Autodesk Inventor part; units mm, degrees
ref_plane "YZ Plane" through (0, 0, 0) normal (1, 0, 0) x (0, 1, 0)
ref_plane "XZ Plane" through (0, 0, 0) normal (0, 1, 0) x (-1, 0, 0)
ref_plane "XY Plane" through (0, 0, 0) normal (0, 0, 1) x (1, 0, 0)
sketch "Sketch1" plane through (0, 0, 0) normal (0, 1, 0) x (-1, 0, 0)
  line L0 (0, 0) -> (0, 28)
  line L1 (0, 28) -> (0, 23)
  circle A0 centre (5, 23) radius 1.5
  circle A1 centre (68, 23) radius 1.5
  line L2 (0, 28) -> (71.7701, 28)
  line L3 (71.7701, 28) -> (71.7701, 0)
  line L4 (71.7701, 0) -> (0, 0)
  line L5 (0, 0) -> (0, -28)
  line L6 (0, -28) -> (0, -23)
  line L7 (0, -23) -> (5, -23)
  circle A2 centre (5, -23) radius 1.5
  circle A3 centre (68, -23) radius 1.5
  line L8 (0, -28) -> (71.7701, -28)
  line L9 (71.7701, -28) -> (71.7701, 0)
  dimension "d0" = 28
  dimension "d4" = 3
  dimension "d6" = 3
extrude "Extrusion1" add sketch "Sketch1" along normal blind 3.175
sketch "Sketch2" plane through (0, 3.175, 0) normal (0, 1, 0) x (1, 0, 0)
  line L0 (0, 28) -> (-71.7701, 28)
  line L1 (-10.8543, 28) -> (-10.8543, -28)
  line L2 (-71.7701, -28) -> (0, -28)
  line L3 (-10.8543, -28) -> (-40.8543, -28)
  line L4 (-40.8543, -28) -> (-40.8543, 28)
  line L5 (-40.8543, 28) -> (-10.8543, 28)
  line L6 (-40.8543, -28) -> (-47.2043, -28)
  line L7 (-47.2043, -28) -> (-47.2043, 28)
  line L8 (-40.8543, 28) -> (-47.2043, 28)
  point P0 (0, 0)
  dimension "d9" = 30
  dimension "d10" = 6.35
revolve "Revolution1" add sketch "Sketch2" angle 20 about axis through (-47.2043, 3.175, 28) along (0, 0, 1)
sketch "Sketch3" plane through (-47.2043, 3.175, 28) normal (-0.342, 0.9397, 0) x (0.9397, 0.342, 0)
  line L0 (0, 0) -> (0, 56)
  line L1 (0, 56) -> (6.35, 56)
  line L2 (43.2716, 56) -> (-24.1703, 56)
  line L3 (6.35, 56) -> (6.35, 0)
  line L4 (0, 0) -> (36.35, 0)
  line L5 (-23.0843, 0) -> (0, 0)
  line L6 (6.35, 0) -> (0, 0)
  line L7 (0, 0) -> (0, 56)
  point P0 (43.2716, 28)
  dimension "d12" = 6.35
extrude "Extrusion2" add sketch "Sketch3" along normal blind 44
sketch "Sketch4" plane through (0, 3.175, 0) normal (0, 1, 0) x (1, 0, 0)
  line L0 (-10.8543, 28) -> (-10.8543, -28)
  line L1 (-10.8543, 0) -> (-10.8543, -7.5)
  line L2 (-10.8543, -7.5) -> (-13.8543, -7.5)
  line L3 (-13.8543, -7.5) -> (-13.8543, 0)
  line L4 (-13.8543, 0) -> (-13.8543, 7.5)
  line L5 (-13.8543, 7.5) -> (-10.8543, 7.5)
  line L6 (-10.8543, 7.5) -> (-10.8543, 0)
  point P0 (0, 0)
  dimension "d15" = 7.5
  dimension "d16" = 3
  dimension "d17" = 7.5
extrude "Extrusion3" cut sketch "Sketch4" along normal mid plane 6.35
sketch "Sketch5" plane through (0, 3.175, 0) normal (0, 1, 0) x (1, 0, 0)
  line L0 (0, 28) -> (-10.8543, 28)
  line L1 (0, 28) -> (-53, 28)
  line L2 (0, 28) -> (-71.7701, 28)
  line L3 (-53, 0) -> (-53, 7.5)
  line L4 (-53, 7.5) -> (-56, 7.5)
  line L5 (-56, 7.5) -> (-56, 0)
  line L6 (-56, 0) -> (-56, -7.5)
  line L7 (-56, -7.5) -> (-53, -7.5)
  line L8 (-53, -7.5) -> (-53, 0)
  point P0 (0, 0)
  dimension "d20" = 53
  dimension "d21" = 7.5
  dimension "d22" = 3
  dimension "d23" = 7.5
extrude "Extrusion4" cut sketch "Sketch5" against normal blind 6.35
fillet "Fillet1" radius 3.175 8 edges at (0, 3.175, 0) (-54.7287, 23.8482, 28) (-54.7287, 23.8482, -28) (-62.2532, 44.5215, 0) (-56, 3.175, 0) (-53, 3.175, 0) (-54.5, 3.175, -7.5) (-54.5, 3.175, 7.5)
fillet "Fillet2" radius 1.524 1 edges at (-71.7701, 3.175, 0)
sketch "Sketch6" plane through (-41.2373, 5.3468, 28) normal (0.9397, 0.342, 0) x (0, 0, -1)
  line L0 (0, 44) -> (3.175, 40.825)
  line L1 (52.825, 40.825) -> (56, 44)
  line L2 (0, 44) -> (56, 44)
  point P0 (28, -19.1283)
sketch "Sketch7" plane through (-41.2373, 5.3468, 28) normal (0.9397, 0.342, 0) x (0, 0, -1)
  line L0 (0, -1.1556) -> (0, 44)
  line L1 (0, 0) -> (0, 44)
  line L2 (56, -1.1556) -> (56, 7.8808)
  point P0 (28, -19.1283)
  point P1 (56, 44)
properties part number "_3DPrint"
Can you work these out from the model? Positions are in its coordinate system, mm. A direction names the side the tool comes from. Round coordinates to 2 decimals unless told otherwise and drop trailing zeros. Order: outer loops, then holes, each group sorted by start corner. A loop starts at its lowest first (then second) coordinate and runs counter-clockwise, first axis right, second up.
(1) If I drill on L1, parallel to Z at x = -5, y = 1; L2, parallel to Y at x = -10.5, z = -18.5 (3 decimals); L3, parallel to X at y = 34, z = -3.5, over which ranges is the centre line in solid material (lowest first)?
Results are:
L1: z = -28 to -24.5, -21.5 to 21.5, 24.5 to 28
L2: y = 0 to 3.175
L3: x = -58.42 to -51.67
(2) I'm going to push flat-ended pins straight in: pin 1 (5 mm diameter, centred on y = 4.5, z = -1, fed in from +X); pin 2 (21 mm diameter, centred on x = -53, z = -4, fed in from +Y); pin 3 (5 mm diameter, centred on y = 38.5, z = -18.5, fed in from +X); pin 4 (1.8 mm diameter, centred on x = -68, z = -23, fed in from +Y). Where does each tip first touch, or does it pass through?
Results are:
pin 1: stops at x = -0.71
pin 2: stops at y = 46.69
pin 3: stops at x = -52.39
pin 4: passes through
(3) On a 3-axis mill with a long thin cutter (end or side, diameter ignored), from which of +Z, -Z, +X, -X, +Y, -Y can I reach the whole of each face in a straight line? I mean faces 1 (the face through (-10.854, 2, 0)), 2 (the face through (-52.045, 2.27, 0.149)), 3 (the face through (-12, 6.35, 0)), 4 (the face through (-12, 3, -7.5)), 5 (the face through (-27.339, 10.405, -0.392)). Say none if no direction works.
Results are:
face 1: +Y, -Y
face 2: none
face 3: +X, -Y
face 4: -Y
face 5: +Z, -Z, +Y
(4) If we section it at B-B (z = 23): Count the separate pieces of the cut face and the enclosed holes in it, plus the area to 3 significant figures.
Results are:
separate pieces: 3
enclosed holes: 0
area: 714 mm2
(5) If we section it at A-A (x = -68): Please give me the cut outline in (y, z) (3 decimals), plus the area to 3 significant figures.
Results are:
outline: (0, -28) - (3.175, -28) - (3.175, -24.5) - (0, -24.5) - close; (0, -21.5) - (3.175, -21.5) - (3.175, 21.5) - (0, 21.5) - close; (0, 24.5) - (3.175, 24.5) - (3.175, 28) - (0, 28) - close
area: 159 mm2
(6) If we section it at D-D (x = -36.5): Please give me the cut outline in (y, z), plus the area to 3 significant figures.
Results are:
outline: (0, -28) - (7.07, -28) - (7.07, 28) - (0, 28) - close
area: 396 mm2
(7) We'd pull the mould along Z, two halves only. Please class faces 6 (the face through (-4.805, 1.565, 21.513)), 7 (the face through (-61.08, 43.93, -0.39)), 8 (the face through (-33, 6, 28)): +Z half, -Z half, draft (parallel to the pull), parting line (faces both ways), or undercut.
Results are:
face 6: undercut
face 7: draft
face 8: +Z half
